```python
from build123d import *

# Parameters (mm, degrees)
F0_W     = 100
F0_H     = 58
F0_R     = 5.035
F1_DEPTH = 7.5
F2_SIZE  = 1.5


with BuildPart() as f1:
    # F0 (on Front) → F1 (new body, symmetric)
    with BuildSketch(Plane.XZ):
        Rectangle(F0_W, F0_H)
        with Locations((-31, 17)):
            Circle(F0_R, mode=Mode.SUBTRACT)
        with BuildLine():
            ThreePointArc((8.0972829663, 7.9192461182), (8.6964862032, 8.8891237283), (9.3632311248, 9.8138714275))
            ThreePointArc((9.3632311248, 9.8138714275), (9.2720779386, 12.7279220614), (12.1861285725, 12.6367688752))
            ThreePointArc((12.1861285725, 12.6367688752), (13.1108762717, 13.3035137968), (14.0807538818, 13.9027170337))
            ThreePointArc((14.0807538818, 13.9027170337), (15.1116982174, 16.6298315852), (17.7690471406, 15.4304581235))
            ThreePointArc((17.7690471406, 15.4304581235), (18.8785548477, 15.6925644865), (20.0039100722, 15.875))
            ThreePointArc((20.0039100722, 15.875), (22, 18), (23.9960899278, 15.875))
            ThreePointArc((23.9960899278, 15.875), (25.1214451523, 15.6925644865), (26.2309528594, 15.4304581235))
            ThreePointArc((26.2309528594, 15.4304581235), (28.8883017826, 16.6298315852), (29.9192461182, 13.9027170337))
            ThreePointArc((29.9192461182, 13.9027170337), (30.8891237283, 13.3035137968), (31.8138714275, 12.6367688752))
            ThreePointArc((31.8138714275, 12.6367688752), (34.7279220614, 12.7279220614), (34.6367688752, 9.8138714275))
            ThreePointArc((34.6367688752, 9.8138714275), (35.3035137968, 8.8891237283), (35.9027170337, 7.9192461182))
            ThreePointArc((35.9027170337, 7.9192461182), (38.6298315852, 6.8883017826), (37.4304581235, 4.2309528594))
            ThreePointArc((37.4304581235, 4.2309528594), (37.6925644865, 3.1214451523), (37.875, 1.9960899278))
            ThreePointArc((37.875, 1.9960899278), (40, 0), (37.875, -1.9960899278))
            ThreePointArc((37.875, -1.9960899278), (37.6925644865, -3.1214451523), (37.4304581235, -4.2309528594))
            ThreePointArc((37.4304581235, -4.2309528594), (38.6298315852, -6.8883017826), (35.9027170337, -7.9192461182))
            ThreePointArc((35.9027170337, -7.9192461182), (35.3035137968, -8.8891237283), (34.6367688752, -9.8138714275))
            ThreePointArc((34.6367688752, -9.8138714275), (34.7279220614, -12.7279220614), (31.8138714275, -12.6367688752))
            ThreePointArc((31.8138714275, -12.6367688752), (30.8891237283, -13.3035137968), (29.9192461182, -13.9027170337))
            ThreePointArc((29.9192461182, -13.9027170337), (28.8883017826, -16.6298315852), (26.2309528594, -15.4304581235))
            ThreePointArc((26.2309528594, -15.4304581235), (25.1214451523, -15.6925644865), (23.9960899278, -15.875))
            ThreePointArc((23.9960899278, -15.875), (22, -18), (20.0039100722, -15.875))
            ThreePointArc((20.0039100722, -15.875), (18.8785548477, -15.6925644865), (17.7690471406, -15.4304581235))
            ThreePointArc((17.7690471406, -15.4304581235), (15.1116982174, -16.6298315852), (14.0807538818, -13.9027170337))
            ThreePointArc((14.0807538818, -13.9027170337), (13.1108762717, -13.3035137968), (12.1861285725, -12.6367688752))
            ThreePointArc((12.1861285725, -12.6367688752), (9.2720779386, -12.7279220614), (9.3632311248, -9.8138714275))
            ThreePointArc((9.3632311248, -9.8138714275), (8.6964862032, -8.8891237283), (8.0972829663, -7.9192461182))
            ThreePointArc((8.0972829663, -7.9192461182), (5.3701684148, -6.8883017826), (6.5695418765, -4.2309528594))
            ThreePointArc((6.5695418765, -4.2309528594), (6.3074355135, -3.1214451523), (6.125, -1.9960899278))
            ThreePointArc((6.125, -1.9960899278), (4, 0), (6.125, 1.9960899278))
            ThreePointArc((6.125, 1.9960899278), (6.3074355135, 3.1214451523), (6.5695418765, 4.2309528594))
            ThreePointArc((6.5695418765, 4.2309528594), (5.3701684148, 6.8883017826), (8.0972829663, 7.9192461182))
        make_face(mode=Mode.SUBTRACT)
    extrude(amount=F1_DEPTH, both=True)

    # F2
    f2_edges = [f1.edges().sort_by_distance(p)[0] for p in [
        (50, 0, 29),
        (0, 7.5, 29),
        (0, -7.5, 29),
        (50, -7.5, 0),
        (50, 7.5, 0),
        (-50, 0, 29),
    ]]
    chamfer(f2_edges, length=F2_SIZE)


solid = f1.part
```
Here's how the part is built. I have some questions about the finished solid (model axes, mm). Give positions to 0.01 mm unless a question says otherwise; leave off trailing zeros. Loops run counter-clockwise (first coordinate to the right, second up) from the corner with the lowest first, then second, coordinate; pieces in that order, holes last. Notation, with made-up numbers: M -14,-26 L 19,-26 A13 ccw 19,-1 Z; hole C 26.5,84.25 d2. An arc over 180 degrees is marked long. Return JSON: item names as keys, results as strings.
Item 1: Please list where these lines run through material, in increasing order: line 1 (Z direction, x = -31, y = 2.25) (3 decimals); line 2 (X direction, y = -5.75, z = -16); line 3 (X direction, y = 2, z = 1).
A:
{"line 1": "z = -29 to 11.965, 22.035 to 29", "line 2": "x = -50 to 14.29, 17.46 to 20, 24 to 26.54, 29.71 to 50", "line 3": "x = -50 to 4.27, 39.73 to 50"}
Item 2: Imagine slicing it at B-B on x = -31. List the corners of the cut face in (y, z) for me (3 decimals).
A:
{"outline": "M -7.5,-29 L 7.5,-29 L 7.5,11.965 L -7.5,11.965 Z; M -7.5,22.035 L 7.5,22.035 L 7.5,27.5 L 6,29 L -6,29 L -7.5,27.5 Z"}
Item 3: Imagine slicing it at A-A on z = 0. List the corners of the cut face in (x, y) for me, then the cut area to 3 significant figures.
A:
{"outline": "M -50,-7.5 L 4,-7.5 L 4,7.5 L -50,7.5 Z; M 40,-7.5 L 48.5,-7.5 L 50,-6 L 50,6 L 48.5,7.5 L 40,7.5 Z", "area": "958 mm^2"}
Item 4: Imagine slicing it at C-C on y = 2.5. State how many separate pieces and enclosed holes the cut face has, then the cut area to 3 significant figures.
A:
{"separate pieces": "1", "enclosed holes": "2", "area": "4,810 mm^2"}
Item 5: Thinking about a two-plate mould opening in X: for faces 1 (the flat face through (-1, 0, 29)), 2 (the flat face through (50, 0, -1)), 3 (the cylindrical face through (40, 0, 0)), which applies, released by +X, released by -X, zero draft, split by the parting line, or undercut?
A:
{"face 1": "zero draft", "face 2": "released by +X", "face 3": "undercut"}
